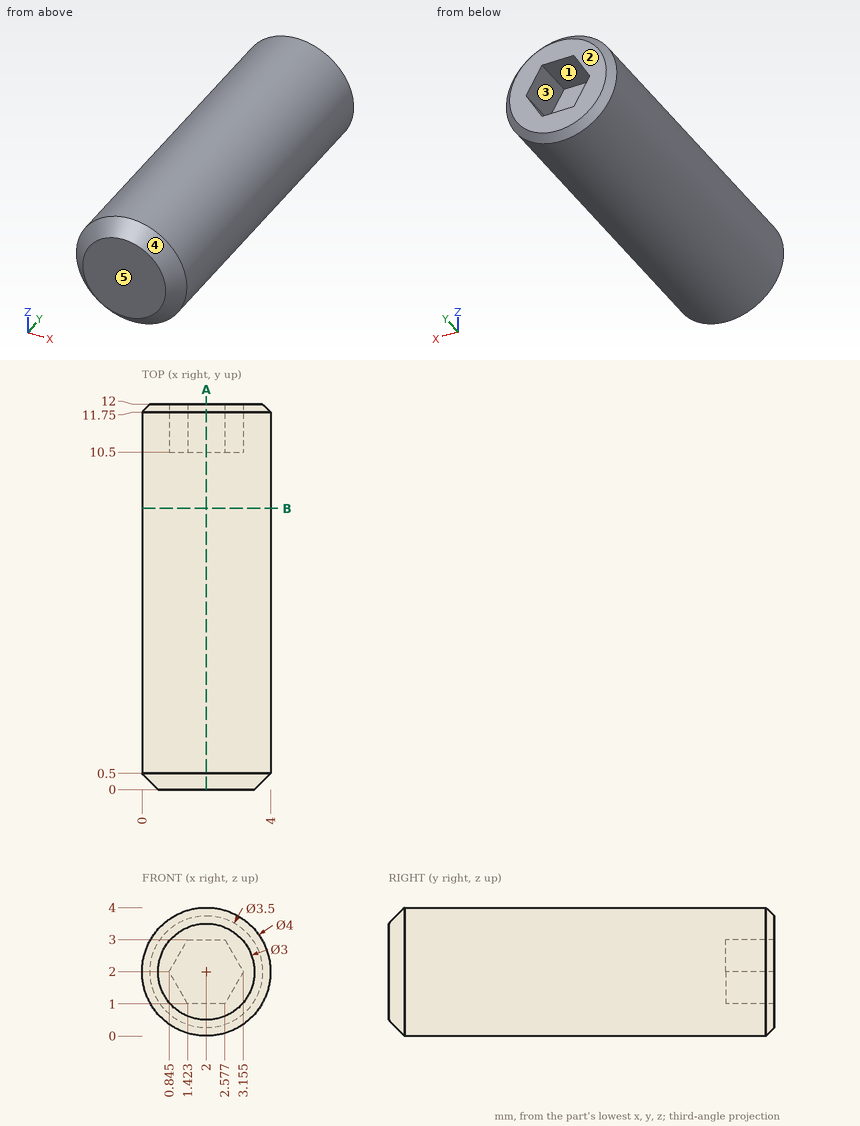
Could you check a few things on this drawing? It's one solid part, dimensions in mm from its lowest x, y, z. A direction names the side the tool comes from. Give positions to 0.01 mm unless a question says otherwise; leave off trailing zeros. Loops run counter-clockwise (first coordinate to the right, second up) from the corner with the lowest first, then second, coordinate; pieces in that order, holes last. Notation, with made-up numbers: M 17.5,18.5 L 53.5,18.5 A13 ccw 53.5,37.5 Z; hole C 4.5,43 d11. An arc over 180 degrees is marked long. Return JSON: item names as keys, results as strings.
Item 1: Please list where these lines run through material, in increasing order: line 1 (X direction, y = 1.5, z = 1.1) (1 decimal); line 2 (Z direction, x = 0.5, y = 2) (1 decimal); line 3 (Z direction, x = 0.35, y = 9.25).
A:
{"line 1": "x = 0.2 to 3.8", "line 2": "z = 0.7 to 3.3", "line 3": "z = 0.87 to 3.13"}
Item 2: Imagine slicing it at B-B on y = 8.75. List the corners of the cut face in (x, z) for me.
A:
{"outline": "C 2,2 d4"}
Item 3: Imagine slicing it at A-A on x = 2. List the corners of the cut face in (y, z) for me, then the cut area to 3 significant figures.
A:
{"outline": "M 0,0.5 L 0.5,0 L 11.75,0 L 12,0.25 L 12,1 L 10.5,1 L 10.5,3 L 12,3 L 12,3.75 L 11.75,4 L 0.5,4 L 0,3.5 Z", "area": "44.7 mm^2"}
Item 4: Thinking about a two-plate mould opening in X: for the marked faces 3, 4 and 5, which applies, released by +X, released by -X, zero draft, split by the parting line, or undercut?
A:
{"face 3": "undercut", "face 4": "split by the parting line", "face 5": "zero draft"}
Item 5: On a 3-axis mill with a long thin cutter (end or side, diameter ignored), from which of +Z, -Z, +X, -X, +Y, -Y can I reach the whole of each face in a straight line? I mean the marked faces 1 and 2. Say none if no direction works.
A:
{"face 1": "+Y", "face 2": "+Z, -Z, +X, -X, +Y"}
